Geometry: final body of the model. Coordinates: model frame, mm. A direction names the side the tool comes from. Coordinates: 2 decimals unless noted, no trailing zeros. Order: outer loops, then holes, each group sorted by start corner. A loop starts at its lowest first (then second) coordinate and runs counter-clockwise, first axis right, second up. Notation, with made-up numbers: M 11.5,72.5 L 57.5,72.5 A14 cw 57.5,97.5 Z; hole C -36.5,16.5 d6. An arc over 180 degrees is marked long. Write item = value, one per line. Start each with the question number.
```python
from build123d import *

# Parameters (mm, degrees)
EXTRUDE_1_DEPTH = 6
SKETCH_2_W      = 13.679492917
SKETCH_2_H      = 41.038478751
SKETCH_2_R      = 2.5
EXTRUDE_2_DEPTH = 2


with BuildPart() as part:
    # 草圖1 → 填料-伸長1 (new body)
    with BuildSketch(Plane.XY):
        with BuildLine():
            Line((8, -24.934633195), (8, 17.94275172))
            ThreePointArc((8, 17.94275172), (0, 25.94275172), (-8, 17.94275172))
            Line((-8, 17.94275172), (-8, -18.141285654))
            Line((-8, -18.141285654), (-8, -24.934633195))
            Line((-8, -24.934633195), (-8, -28.206652459))
            Line((-8, -28.206652459), (-8, -35))
            Line((-8, -35), (-3, -35))
            Line((-3, -35), (-3, -45))
            ThreePointArc((-3, -45), (4.367409356, -37.826519096), (8, -28.206652459))
            Line((8, -28.206652459), (8, -24.934633195))
        make_face()
        with BuildLine():
            ThreePointArc((-4.999271035, -4.154189345), (-6.5, 0), (-4.999271035, 4.154189345))
            Line((-4.999271035, 4.154189345), (-2.6, 17.94275172))
            ThreePointArc((-2.6, 17.94275172), (0, 20), (2.6, 17.94275172))
            Line((2.6, 17.94275172), (4.999271035, 4.154189345))
            ThreePointArc((4.999271035, 4.154189345), (6.5, 0), (4.999271035, -4.154189345))
            Line((4.999271035, -4.154189345), (2.6, -17.94275172))
            ThreePointArc((2.6, -17.94275172), (0, -20), (-2.6, -17.94275172))
            Line((-2.6, -17.94275172), (-4.999271035, -4.154189345))
        make_face(mode=Mode.SUBTRACT)
    extrude(amount=EXTRUDE_1_DEPTH)

    # 草圖2 → 填料-伸長2 (add)
    with BuildSketch(Plane.XY):
        with Locations((0.193072501, -0.109084802)):
            Rectangle(SKETCH_2_W, SKETCH_2_H)
        Circle(SKETCH_2_R, mode=Mode.SUBTRACT)
    extrude(amount=EXTRUDE_2_DEPTH)


solid = part.part
```
Item 1: Section query B-B on y = 0. Output: boundary loops of the cut face in (x, z).
Item 2: Material intervals for probe 1 along X at (y, z) = (-9, 5.7); probe 2 along Z at (x, y) = (2.5, 18); probe 3 along Y at (x, z) = (1.5, 3), sorted ascending. Write a range as [from, to].
Item 3: Section query C-C on x = 0. Output: boundary loops of the cut face in (y, z), and give its area (3 significant figures).
Item 4: Draft query along X for faces 1 (the cylindrical face through (4.288, -37.948, 2.958)), 2 (the cylindrical face through (0.18, 25.94, 2.96)), 3 (the flat face through (3, 0, 2)), 4 (the flat face through (-5, -9, 6)). Return one class per face: pulls with the +X half, pulls with the -X half, needs draft (parallel to the pull), parting line crosses it, or undercut.
Item 5: First-contact query: pin 1 (3 mm diameter, centred on x = 0, y = 0, fed in from +Z); pin 2 (1.8 mm diameter, centred on y = -40, z = 3, fed in from -X). Flat tips, straight axial feed; report the tip coordinate or a pass-through.
Item 6: Reachability of faces 5 (the flat face through (-3.783, -11.145, 3.972)), 6 (the flat face through (-3, -40, 3)), 7 (the flat face through (0, -9, 0)) from +Z, -Z, +X, -X, +Y, -Y: full face, straight path, thin tool, end or side. Return the list, or none.
Item 7: Section query A-A on z = 1.4. Output: boundary loops of the cut face in (x, y), and give its area (3 significant figures).
Item 8: Section query D-D on y = -16.5. Output: boundary loops of the cut face in (x, z), and give its area (3 significant figures).
Ans:
q1.outline = M -8,0 L -2.5,0 L -2.5,2 L -6.5,2 L -6.5,6 L -8,6 Z; M 2.5,0 L 8,0 L 8,6 L 6.5,6 L 6.5,2 L 2.5,2 Z
q2.probe_1 = [-8, -4.16], [4.16, 8]
q2.probe_2 = [0, 2]
q2.probe_3 = [-41.4, -19.54], [19.54, 25.8]
q3.outline = M -42.8,0 L -2.5,0 L -2.5,2 L -20,2 L -20,6 L -42.8,6 Z; M 2.5,0 L 25.94,0 L 25.94,6 L 20,6 L 20,2 L 2.5,2 Z
q3.area = 242 mm^2
q4.face_1 = pulls with the +X half
q4.face_2 = parting line crosses it
q4.face_3 = undercut
q4.face_4 = needs draft
q5.pin_1 = through
q5.pin_2 = -3
q6.face_5 = +Z
q6.face_6 = +Z, -Z, -X, -Y
q6.face_7 = -Z, +X, -X, +Y, -Y
q7.outline = M -8,-35 L -3,-35 L -3,-45 A23.68 ccw 8,-28.21 L 8,17.94 A8 ccw -8,17.94 Z; hole C 0,0 d5
q7.area = 976 mm^2
q8.outline = M -8,0 L 8,0 L 8,6 L 2.85,6 L 2.85,2 L -2.85,2 L -2.85,6 L -8,6 Z
q8.area = 73.2 mm^2
